The model under review builds one solid part; all positions refer to its coordinate system, in mm. Face numbers are marked on the shaded views. Coordinates: 2 decimals unless noted, no trailing zeros. Order: outer loops, then holes, each group sorted by start corner. A loop starts at its lowest first (then second) coordinate and runs counter-clockwise, first axis right, second up. Notation, with made-up numbers: (74.5, -34) -> (105.5, -34) arc R30 cw to (105.5, -6) -> close; hole circle Ø5 at (20, 76.5). An arc over 180 degrees is marked (long way). Use one line per item in the form item = value.
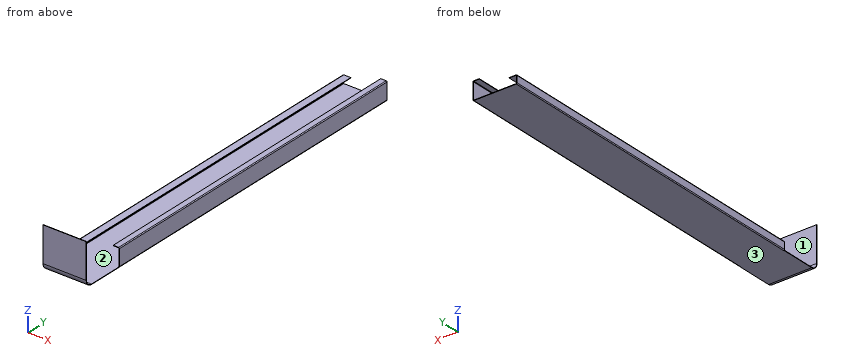
from build123d import *

# Parameters (mm, degrees)
BASE_FLANGE1_DEPTH = 814
EDGE_FLANGE1_DEPTH = 814
SKETCH15_W         = 104
SKETCH15_H         = 84
TAB1_DEPTH         = 1
EDGE_FLANGE2_DEPTH = 104


# Sheet-metal steps are written as plain solids
with BuildPart() as part:
    # Sketch1 → Base-Flange1 (new body)
    with BuildSketch(Plane(origin=(0, 0, 0), x_dir=(1, 0, 0), z_dir=(0, 1, 0))):
        with BuildLine():
            Line((104, 18.695652174), (104, 57.695652174))
            ThreePointArc((104, 57.695652174), (103.707106781, 58.402758955), (103, 58.695652174))
            Line((103, 58.695652174), (1, 58.695652174))
            ThreePointArc((1, 58.695652174), (0.292893219, 58.402758955), (0, 57.695652174))
            Line((0, 57.695652174), (0, 41.695652174))
            ThreePointArc((0, 41.695652174), (0.292893219, 40.988545393), (1, 40.695652174))
            Line((1, 40.695652174), (18, 40.695652174))
            Line((18, 40.695652174), (18, 39.695652174))
            Line((18, 39.695652174), (1, 39.695652174))
            ThreePointArc((1, 39.695652174), (-0.414213562, 40.281438612), (-1, 41.695652174))
            Line((-1, 41.695652174), (-1, 57.695652174))
            ThreePointArc((-1, 57.695652174), (-0.414213562, 59.109865736), (1, 59.695652174))
            Line((1, 59.695652174), (103, 59.695652174))
            ThreePointArc((103, 59.695652174), (104.414213562, 59.109865736), (105, 57.695652174))
            Line((105, 57.695652174), (105, 18.695652174))
            Line((105, 18.695652174), (104, 18.695652174))
        make_face()
    extrude(amount=BASE_FLANGE1_DEPTH)

    # Edge-Flange1 section (across the edge) → Edge-Flange1 (add)
    with BuildSketch(Plane(origin=(104, 0, -17.695652174), x_dir=(0, 0, -1), z_dir=(0, 1, 0))):
        with BuildLine():
            Line((-1, 1), (-1, 14))
            Line((-1, 14), (0, 14))
            Line((0, 14), (0, 1))
            ThreePointArc((0, 1), (0.292893219, 0.292893219), (1, 0))
            Line((1, 0), (1, -1))
            ThreePointArc((1, -1), (-0.414213562, -0.414213562), (-1, 1))
        make_face()
    extrude(amount=EDGE_FLANGE1_DEPTH)

    # Sketch15 → Tab1 (add)
    with BuildSketch(Plane(origin=(0, 0, -59.695652174), x_dir=(-1, 0, 0), z_dir=(0, 0, -1))):
        with Locations((-52, -42)):
            Rectangle(SKETCH15_W, SKETCH15_H)
    extrude(amount=-TAB1_DEPTH)

    # Edge-Flange2 section (across the edge) → Edge-Flange2 (add)
    with BuildSketch(Plane(origin=(0, -99, -58.695652174), x_dir=(0, 1, 0), z_dir=(1, 0, 0))):
        with BuildLine():
            Line((-1, 15), (-1, 99))
            Line((-1, 99), (0, 99))
            Line((0, 99), (0, 15))
            ThreePointArc((0, 15), (4.393398282, 4.393398282), (15, 0))
            Line((15, 0), (15, -1))
            ThreePointArc((15, -1), (3.686291501, 3.686291501), (-1, 15))
        make_face()
    extrude(amount=EDGE_FLANGE2_DEPTH)


solid = part.part
Item 1: Clearance check with flat-ended pins moving along their axes: pin 1 (4 mm diameter, centred on x = 16.5, y = 610.5, fed in from +Z); pin 2 (10.5 mm diameter, centred on x = 97, y = 222.5, fed in from +Z); pin 3 (1.1 mm diameter, centred on y = 438, z = -17.5, fed in from -X). State where each tip first meets the part, or that it passes through.
Results found:
pin_1 = -39.7
pin_2 = -16.7
pin_3 = 90
Item 2: We need section A-A (z = -29). Write out the cut boundary in (x, y), plus the area to 3 significant figures.
Results found:
outline = (0, -100) -> (104, -100) -> (104, -99) -> (0, -99) -> close; (104, 0) -> (105, 0) -> (105, 814) -> (104, 814) -> close
area = 918 mm²
Item 3: Draft analysis for pull direction Z (two halves, no side actions). For the marked faces 1, 2 and 3, state which applies: released by +Z, released by -Z, zero draft, split by the parting line, or undercut.
Results found:
face_1 = zero draft
face_2 = undercut
face_3 = released by -Z
Item 4: We need section B-B (y = 678.5). Write out the cut boundary in (x, z).
Results found:
outline = (-1, -57.7) arc R2 ccw to (1, -59.7) -> (103, -59.7) arc R2 ccw to (105, -57.7) -> (105, -18.7) arc R2 ccw to (103, -16.7) -> (90, -16.7) -> (90, -17.7) -> (103, -17.7) arc R1 cw to (104, -18.7) -> (104, -57.7) arc R1 cw to (103, -58.7) -> (1, -58.7) arc R1 cw to (0, -57.7) -> (0, -41.7) arc R1 cw to (1, -40.7) -> (18, -40.7) -> (18, -39.7) -> (1, -39.7) arc R2 ccw to (-1, -41.7) -> close
Item 5: We need section D-D (z = 6). Write out the cut boundary in (x, y), plus the area to 3 significant figures.
Results found:
outline = (0, -100) -> (104, -100) -> (104, -99) -> (0, -99) -> close
area = 104 mm²
Item 6: To check wall thickness, follow L1, parallel to Z at x = 99.5, y = 184; L2, parallel to Z at x = 78.5, y = 433; L3, parallel to Y at x = 50.5, z = -29.5. State the ranges of each line that lie inside material, in increasing order. Write a range as from..to.
Results found:
L1 = -59.7..-58.7, -17.7..-16.7
L2 = -59.7..-58.7
L3 = -100..-99
Item 7: We need section C-C (x = 59). Write out the cut boundary in (y, z).
Results found:
outline = (-100, -43.7) arc R16 ccw to (-84, -59.7) -> (814, -59.7) -> (814, -58.7) -> (-84, -58.7) arc R15 cw to (-99, -43.7) -> (-99, 40.3) -> (-100, 40.3) -> close
